Input: part model. Units: mm. Frame: model coordinates. A direction names the side the tool comes from. Coordinates: 2 decimals unless noted, no trailing zeros. Loops run counter-clockwise (first coordinate to the right, second up) from the corner with the lowest first, then second, coordinate; pieces in that order, holes last.
(1) Section A-A, the plane y = 3.05. Give the number of separate pieces and of enclosed holes in the cut face, then the cut area to 3 significant figures.
(2) Mould query, pull axis X, two halves, no side actions, for faces 4 (the face through (-0.3, 2.5, -5.4)), 5 (the face through (-1, 5, -3)), 6 (the face through (6, 2, 0)). Classes: released by +X, released by -X, zero draft, split by the parting line, or undercut.
(3) Line query: L1, parallel to X at y = 3.75, z = -5; L2, parallel to Z at x = -5.25, y = 2.3. Output: solid intervals per line, ascending.
(4) Contact query for flat-ended pins moving along their axis: P1, Ø1, axis at x = 5, y = 2, coming from the -Z side; P2, Ø2.5, axis at y = 3.5, z = -23.5, coming from the -X side. Output: stop coordinate, or through.
(5) Section B-B, the plane z = -7. Return loops of the section in (x, y).
(6) Set-up query: faces 1 (the face through (2.5, 2, -23)), 2 (the face through (-2.5, 2, -22)), 3 (the face through (-0.3, 2.5, -1.4)). Return all of +Z, -Z, +X, -X, +Y, -Y with unobstructed straight access to the full face (end or side cutting, diameter ignored); none if empty.
```python
from build123d import *

# Parameters (mm, degrees)
SKETCH1_R           = 0.5
BOSS_EXTRUDE1_DEPTH = 5


with BuildPart() as part:
    # Sketch1 → Boss-Extrude1 (new body)
    with BuildSketch(Plane(origin=(0, 0, 0), x_dir=(1, 0, 0), z_dir=(0, 1, 0))):
        Polygon((-2.5, 20), (-2.5, 25), (2.5, 25), (2.5, 20), (6, 20), (6, -20), (-6, -20), (-6, 20), align=None)
        with Locations(Location((0, 11, 0), (0, 0, 270))):
            Circle(SKETCH1_R, mode=Mode.SUBTRACT)
        with Locations(Location((0, 9, 0), (0, 0, 270))):
            Circle(SKETCH1_R, mode=Mode.SUBTRACT)
        with Locations(Location((0, 7, 0), (0, 0, 270))):
            Circle(SKETCH1_R, mode=Mode.SUBTRACT)
        with Locations(Location((0, 5, 0), (0, 0, 270))):
            Circle(SKETCH1_R, mode=Mode.SUBTRACT)
        with Locations(Location((0, 3, 0), (0, 0, 270))):
            Circle(SKETCH1_R, mode=Mode.SUBTRACT)
        with Locations(Location((0, 1, 0), (0, 0, 270))):
            Circle(SKETCH1_R, mode=Mode.SUBTRACT)
        with Locations(Location((0, -7.5, 0), (0, 0, 270))):
            Circle(SKETCH1_R, mode=Mode.SUBTRACT)
        with Locations(Location((0, -9.5, 0), (0, 0, 270))):
            Circle(SKETCH1_R, mode=Mode.SUBTRACT)
        with Locations(Location((0, -11.5, 0), (0, 0, 270))):
            Circle(SKETCH1_R, mode=Mode.SUBTRACT)
        with Locations(Location((0, -13.5, 0), (0, 0, 270))):
            Circle(SKETCH1_R, mode=Mode.SUBTRACT)
        with Locations(Location((0, -15.5, 0), (0, 0, 270))):
            Circle(SKETCH1_R, mode=Mode.SUBTRACT)
        with Locations(Location((0, -17.5, 0), (0, 0, 270))):
            Circle(SKETCH1_R, mode=Mode.SUBTRACT)
    extrude(amount=BOSS_EXTRUDE1_DEPTH)


solid = part.part
```
Report:
1. separate pieces: 1
1. enclosed holes: 12
1. area: 496 mm2
2. face 4: undercut
2. face 5: zero draft
2. face 6: released by +X
3. L1: x = -6 to -0.5, 0.5 to 6
3. L2: z = -20 to 20
4. P1: stops at z = -20
4. P2: stops at x = -2.5
5. outline: (-6, 0) - (-0.5, 0) - (-0.5, 5) - (-6, 5) - close; (0.5, 0) - (6, 0) - (6, 5) - (0.5, 5) - close
6. face 1: -Z, +X, +Y, -Y
6. face 2: -Z, -X, +Y, -Y
6. face 3: +Y, -Y
